```python
from build123d import *

# Parameters (mm, degrees)
SKETCH1_R           = 73.325
SKETCH1_R_2         = 1.65
SKETCH1_R_3         = 2.7
SKETCH1_R_4         = 25
BOSS_EXTRUDE1_DEPTH = 2.5
BOSS_EXTRUDE2_DEPTH = 15
FILLET2_R           = 4
CUT_EXTRUDE1_DEPTH  = 105.776482333
FILLET1_R           = 4


with BuildPart() as part:
    # Sketch1 → Boss-Extrude1 (new body)
    with BuildSketch(Plane.XY):
        Circle(SKETCH1_R)
        with Locations((0, 68.825)):
            Circle(SKETCH1_R_2, mode=Mode.SUBTRACT)
        with Locations((-68.825, 0)):
            Circle(SKETCH1_R_3, mode=Mode.SUBTRACT)
        Circle(SKETCH1_R_4, mode=Mode.SUBTRACT)
        with Locations((0, -68.825)):
            Circle(SKETCH1_R_2, mode=Mode.SUBTRACT)
        with Locations((68.825, 0)):
            Circle(SKETCH1_R_3, mode=Mode.SUBTRACT)
        with BuildLine():
            Line((-37.5, 8.75), (-37.5, -8.75))
            ThreePointArc((-37.5, -8.75), (-39.55, -10.8), (-41.6, -8.75))
            Line((-41.6, -8.75), (-41.6, 8.75))
            ThreePointArc((-41.6, 8.75), (-39.55, 10.8), (-37.5, 8.75))
        make_face(mode=Mode.SUBTRACT)
        with BuildLine():
            Line((10, -41.35), (-10, -41.35))
            ThreePointArc((-10, -41.35), (-12.05, -39.3), (-10, -37.25))
            Line((-10, -37.25), (10, -37.25))
            ThreePointArc((10, -37.25), (12.05, -39.3), (10, -41.35))
        make_face(mode=Mode.SUBTRACT)
        with BuildLine():
            Line((41.6, -8.75), (41.6, 8.75))
            ThreePointArc((41.6, 8.75), (39.55, 10.8), (37.5, 8.75))
            Line((37.5, 8.75), (37.5, -8.75))
            ThreePointArc((37.5, -8.75), (39.55, -10.8), (41.6, -8.75))
        make_face(mode=Mode.SUBTRACT)
        with BuildLine():
            Line((-6, 58.1), (6, 58.1))
            ThreePointArc((6, 58.1), (8.05, 56.05), (6, 54))
            Line((6, 54), (-6, 54))
            ThreePointArc((-6, 54), (-8.05, 56.05), (-6, 58.1))
        make_face(mode=Mode.SUBTRACT)
    extrude(amount=BOSS_EXTRUDE1_DEPTH)

    # Sketch2 → Boss-Extrude2 (add)
    with BuildSketch(Plane.XY.offset(2.5)):
        with BuildLine():
            Line((-26.69328099, 26.69328099), (-28.814601333, 28.814601333))
            ThreePointArc((-28.814601333, 28.814601333), (0, 40.75), (28.814601333, 28.814601333))
            Line((28.814601333, 28.814601333), (26.69328099, 26.69328099))
            ThreePointArc((26.69328099, 26.69328099), (0, 37.75), (-26.69328099, 26.69328099))
        make_face()
    extrude(amount=BOSS_EXTRUDE2_DEPTH)

    # Fillet2
    fillet2_edges = [part.edges().sort_by_distance(p)[0] for p in [
        (0, 37.75, 2.5),
        (27.753941162, 27.753941162, 2.5),
        (0, 40.75, 2.5),
        (-27.753941162, 27.753941162, 2.5),
    ]]
    fillet(fillet2_edges, radius=FILLET2_R)

    # Sketch4 → Cut-Extrude1 (cut, through all)
    with BuildSketch(Plane.XY.offset(2.5)):
        with BuildLine():
            Line((71.976076755, 14), (53.188344588, 14))
            ThreePointArc((53.188344588, 14), (38.890872965, 38.890872965), (14, 53.188344588))
            Line((14, 53.188344588), (14, 71.976076755))
            ThreePointArc((14, 71.976076755), (51.848604731, 51.848604731), (71.976076755, 14))
        make_face()
        with BuildLine():
            Line((-71.976076755, -14), (-53.188344588, -14))
            ThreePointArc((-53.188344588, -14), (-38.890872965, -38.890872965), (-14, -53.188344588))
            Line((-14, -53.188344588), (-14, -71.976076755))
            ThreePointArc((-14, -71.976076755), (-51.848604731, -51.848604731), (-71.976076755, -14))
        make_face()
        with BuildLine():
            Line((71.976076755, -14), (53.188344588, -14))
            ThreePointArc((53.188344588, -14), (38.890872965, -38.890872965), (14, -53.188344588))
            Line((14, -53.188344588), (14, -71.976076755))
            ThreePointArc((14, -71.976076755), (51.848604731, -51.848604731), (71.976076755, -14))
        make_face()
        with BuildLine():
            Line((-71.976076755, 14), (-53.188344588, 14))
            ThreePointArc((-53.188344588, 14), (-38.890872965, 38.890872965), (-14, 53.188344588))
            Line((-14, 53.188344588), (-14, 71.976076755))
            ThreePointArc((-14, 71.976076755), (-51.848604731, 51.848604731), (-71.976076755, 14))
        make_face()
    extrude(amount=-CUT_EXTRUDE1_DEPTH, mode=Mode.SUBTRACT)

    # Fillet1
    fillet1_edges = [part.edges().sort_by_distance(p)[0] for p in [
        (-14, 53.188344588, 1.25),
        (-53.188344588, 14, 1.25),
        (-71.976076755, 14, 1.25),
        (-14, 71.976076755, 1.25),
        (14, 71.976076755, 1.25),
        (71.976076755, 14, 1.25),
        (53.188344588, 14, 1.25),
        (14, 53.188344588, 1.25),
        (14, -53.188344588, 1.25),
        (53.188344588, -14, 1.25),
        (71.976076755, -14, 1.25),
        (14, -71.976076755, 1.25),
        (-14, -71.976076755, 1.25),
        (-71.976076755, -14, 1.25),
        (-53.188344588, -14, 1.25),
        (-14, -53.188344588, 1.25),
    ]]
    fillet(fillet1_edges, radius=FILLET1_R)


solid = part.part
```
The model under review builds one solid part; all positions refer to its coordinate system, in mm. A direction names the side the tool comes from. Round coordinates to 2 decimals unless told otherwise and drop trailing zeros. Loops run counter-clockwise (first coordinate to the right, second up) from the corner with the lowest first, then second, coordinate; pieces in that order, holes last. Notation, with made-up numbers: (-8, 8.5) - (30, 8.5) arc R18 ccw to (30, 41.5) - close; hole circle Ø6 at (80.5, -11). An arc over 180 degrees is marked (long way). Use a Markdown table: item, result. Add a question column.
Q1. Add section A-A (y = -21). State the section outline as (x, z) points.
Q2. Add section B-B (x = -39.55). State the section outline as (y, z) points, plus the area to 3 significant figures.
Q3. For probe 1 along Y at (x, z) = (0, 1.65) (3 decimals); probe 2 along Z at (x, y) = (35, -26); probe 3 along Y at (x, z) = (56, 1.5), list the stretches that pass through material, from the lowest coordinate up.
Q4. Add section C-C (z = 15.25). State the section outline as (x, y) points, plus the area to 3 significant figures.
Q5. Add section D-D (x = 46.5). State the section outline as (y, z) points.
Q6. The part is to be moulded in two halves that separate along Y. For faces 3 (the face through (0.415, 37.748, 11.923)), 4 (the face through (-39.15, 38.63, 1.27)), 5 (the face through (-0.358, -70.436, 1.232)), say which applies: pulls with the +Y half, pulls with the -Y half, needs draft (parallel to the pull), parting line crosses it, or undercut.
Q7. Machinability: for faces 1 (the face through (39.15, -38.63, 1.27)), 2 (the face through (-0.448, 40.748, 11.923)), which of the approach directions +Z, -Z, +X, -X, +Y, -Y give a long, thin tool a straight path to every point of the face, cutting with its end or side? Answer none if there is none.
Q8. Insertion check: pin 1 Ø1.2 at (x, z) = (-61.5, 2) entering from +Y; pin 2 Ø0.8 at (x, z) = (-60.5, 1.5) entering from -Y; pin 3 Ø0.8 at (y, z) = (3, 1) entering from +X. Each pin has a flat end and moves straight along its axis. Give the tip position at first contact, or say it passes through.
Worked answers:
| question | item | result |
|---|---|---|
| 1 | outline | (-50.83, 0) - (-13.56, 0) - (-13.56, 2.5) - (-50.83, 2.5) - close; (13.56, 0) - (50.83, 0) - (50.83, 2.5) - (13.56, 2.5) - close |
| 2 | outline | (-38.22, 0) - (-10.8, 0) - (-10.8, 2.5) - (-38.22, 2.5) - close; (10.8, 0) - (38.22, 0) - (38.22, 2.5) - (10.8, 2.5) - close |
| 2 | area | 137 mm² |
| 3 | probe 1 | -73.325 to -70.475, -67.175 to -41.35, -37.25 to -25, 25 to 54, 58.1 to 67.175, 70.475 to 73.325 |
| 3 | probe 2 | 0 to 2.5 |
| 3 | probe 3 | -14 to 14 |
| 4 | outline | (-28.81, 28.81) - (-26.69, 26.69) arc R37.75 cw to (26.69, 26.69) - (28.81, 28.81) arc R40.75 ccw to start |
| 4 | area | 185 mm² |
| 5 | outline | (-29.37, 0) - (29.37, 0) - (29.37, 2.5) - (-29.37, 2.5) - close |
| 6 | face 3 | pulls with the -Y half |
| 6 | face 4 | pulls with the +Y half |
| 6 | face 5 | undercut |
| 7 | face 1 | +Z, -Z, +X, -Y |
| 7 | face 2 | +Z, +Y |
| 8 | pin 1 | y = 14 |
| 8 | pin 2 | y = -14 |
| 8 | pin 3 | x = 73.28 |
